The drawing under review shows one solid part. Ordinate dimensions are in mm from its lowest x, y, z. A direction names the side the tool comes from. Coordinates: 2 decimals unless noted, no trailing zeros. Order: outer loops, then holes, each group sorted by start corner. A loop starts at its lowest first (then second) coordinate and runs counter-clockwise, first axis right, second up.
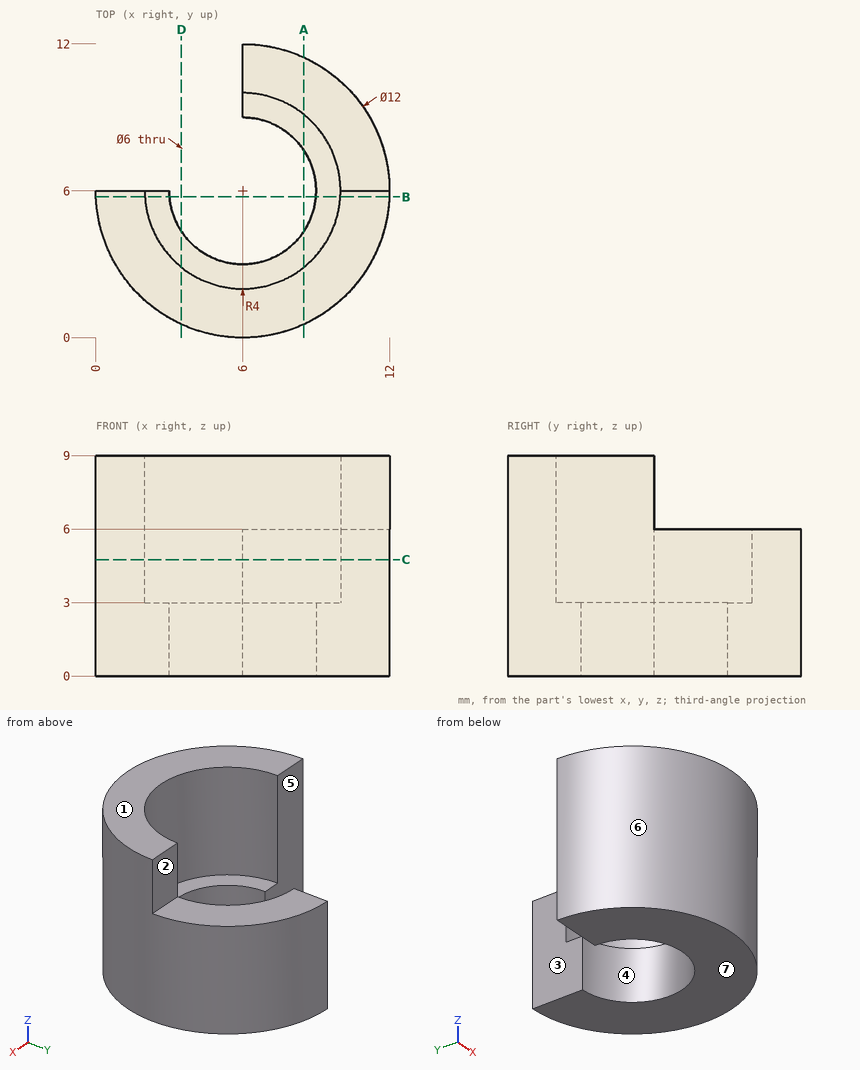
1. Take a section at A-A, the plane x = 8.5. Give the boundary of the cut face in (y, z).
Answer below:
outline: (0.55, 0) - (4.34, 0) - (4.34, 3) - (2.88, 3) - (2.88, 9) - (0.55, 9) - close; (7.66, 0) - (11.45, 0) - (11.45, 6) - (9.12, 6) - (9.12, 3) - (7.66, 3) - close
2. To check wall thickness, follow L1, parallel to Z at x = 2.75, y = 5; L2, parallel to Y at x = 7.75, z = 1.75; L3, parallel to X at y = 5.25, z = 7.25. State the ranges of each line that lie inside material, in increasing order.
Answer below:
L1: z = 0 to 3
L2: y = 0.26 to 3.56, 8.44 to 11.74
L3: x = 0.05 to 2.07, 9.93 to 11.95
3. Machinability: for the marked faces 1, 2 and 3, which of the approach directions +Z, -Z, +X, -X, +Y, -Y give a long, thin tool a straight path to every point of the face, cutting with its end or side? Answer none if there is none.
Answer below:
face 1: +Z, +X, -X, +Y, -Y
face 2: +Z, +X, -X, +Y
face 3: +Z, -Z, -X, +Y
4. Clearance check with flat-ended pins moving along their axes: pin 1 Ø5 at (x, z) = (10.5, 5.5) entering from +Y; pin 2 Ø2.5 at (y, z) = (11, 3.5) entering from -X; pin 3 Ø1 at (x, z) = (10, 1) entering from -Y. State where each tip first meets the part, or that it passes through.
Answer below:
pin 1: stops at y = 11.66
pin 2: stops at x = 6
pin 3: stops at y = 1.13
5. Take a section at C-C, the plane z = 4.75. Give the boundary of the cut face in (x, y).
Answer below:
outline: (0, 6) arc R6 ccw (long way) to (6, 12) - (6, 10) arc R4 cw (long way) to (2, 6) - close
6. Take a section at B-B, the plane y = 5.75. Give the boundary of the cut face in (x, z).
Answer below:
outline: (0.01, 0) - (3.01, 0) - (3.01, 3) - (2.01, 3) - (2.01, 9) - (0.01, 9) - close; (8.99, 0) - (11.99, 0) - (11.99, 9) - (9.99, 9) - (9.99, 3) - (8.99, 3) - close
7. The part is to be moulded in two halves that separate along Y. For the marked faces 4, 5, 6 and 7, say which applies: +Y half, -Y half, draft (parallel to the pull), parting line (faces both ways), or undercut.
Answer below:
face 4: undercut
face 5: +Y half
face 6: parting line
face 7: draft
8. Take a section at D-D, the plane x = 3.5. Give the boundary of the cut face in (y, z), plus the area to 3 significant figures.
Answer below:
outline: (0.55, 0) - (4.34, 0) - (4.34, 3) - (2.88, 3) - (2.88, 9) - (0.55, 9) - close
area: 25.4 mm2
